from build123d import *

# Parameters (mm, degrees)
SKETCH2_R          = 1.8288
CUT_EXTRUDE1_DEPTH = 43.573973945


with BuildPart() as part:
    # Sketch1 → Revolve1 (revolve)
    with BuildSketch(Plane(origin=(0, 0, 0), x_dir=(1, 0, 0), z_dir=(0, 1, 0))):
        with BuildLine():
            Line((7.9629, -25.4), (44.45, -25.4))
            Line((44.45, -25.4), (44.45, 0))
            Line((44.45, 0), (46.99, 0))
            Line((46.99, 0), (58.473357526, 14.633973945))
            Line((58.473357526, 14.633973945), (48.488896002, -2.93998396))
            ThreePointArc((48.488896002, -2.93998396), (47.371046022, -5.678922959), (46.99, -8.612551998))
            Line((46.99, -8.612551998), (46.99, -27.94))
            Line((46.99, -27.94), (0, -27.94))
            Line((0, -27.94), (0, -15.24))
            Line((0, -15.24), (5.4229, -15.24))
            Line((5.4229, -15.24), (7.9629, -17.78))
            Line((7.9629, -17.78), (7.9629, -25.4))
        make_face()
    revolve(axis=Axis((0, 0, 0), (0, 0, 1)))

    # Sketch2 → Cut-Extrude1 (cut, through all)
    with BuildSketch(Plane.XY.offset(27.94)):
        with Locations((0, 16)):
            Circle(SKETCH2_R)
        with Locations((15.216904261, 4.94427191)):
            Circle(SKETCH2_R)
        with Locations((9.404564037, -12.94427191)):
            Circle(SKETCH2_R)
        with Locations((-9.404564037, -12.94427191)):
            Circle(SKETCH2_R)
        with Locations((-15.216904261, 4.94427191)):
            Circle(SKETCH2_R)
    extrude(amount=-CUT_EXTRUDE1_DEPTH, mode=Mode.SUBTRACT)


solid = part.part
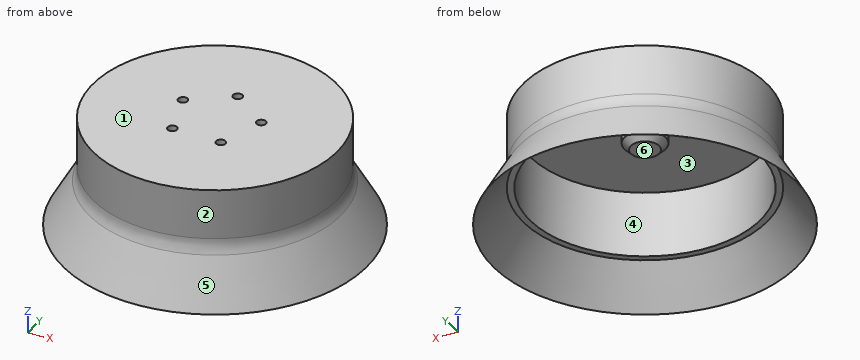
The model under review builds one solid part; all positions refer to its coordinate system, in mm. Face numbers are marked on the shaded views. A direction names the side the tool comes from. Give positions to 0.01 mm unless a question says otherwise; leave off trailing zeros. Loops run counter-clockwise (first coordinate to the right, second up) from the corner with the lowest first, then second, coordinate; pieces in that order, holes last. Notation, with made-up numbers: (63.5, -21) -> (97.5, -21) arc R10 cw to (97.5, -7) -> close; hole circle Ø5 at (81.5, 83). An arc over 180 degrees is marked (long way). Put each result on its own line as item: value. Start each with the question number.
1. Mouldability with a two-part tool opening along Y and no side actions: class the marked faces 1, 2, 3 and 4 as released by +Y, released by -Y, zero draft, split by the parting line, or undercut.
2. Wall thickness on probe 1 along Y at (x, z) = (0, 26); probe 2 along Z at (x, y) = (-25, 27); probe 3 along X at (y, z) = (-10, 9): over which ranges is each line inside the solid? List them lowest first.
3. Clearance check with flat-ended pins moving along their axes: P1, Ø6, axis at x = 2.5, z = -9.5, coming from the -Y side; P2, Ø5.5, axis at x = -1, y = 2, coming from the -Z side; P3, Ø4, axis at x = -7.5, y = -32.5, coming from the -Z side. State where each tip first meets the part, or that it passes through.
4. We need section A-A on x = 0. State the section outline as (y, z) points.
5. For the marked faces 5 and 6, list the 3-axis set-ups (+Z, -Z, +X, -X, +Y, -Y) from which the entire face can be reached by the end or side of a thin tool; tool diameter is ignored.
6. We need section B-B on y = 0. State the section outline as (x, z) points, then the cut area to 3 significant figures.
7. We need section C-C on z = -3. State the section outline as (x, y) points.
Determined:
1. face 1: zero draft
1. face 2: split by the parting line
1. face 3: undercut
1. face 4: undercut
2. probe 1: -46.99 to 14.17, 17.83 to 46.99
2. probe 2: 25.4 to 27.94
2. probe 3: -45.91 to -43.31, 43.31 to 45.91
3. P1: y = -57.21
3. P2: z = 15.24
3. P3: z = 25.4
4. outline: (-58.47, -14.63) -> (-46.99, 0) -> (-44.45, 0) -> (-44.45, 25.4) -> (-7.96, 25.4) -> (-7.96, 17.78) -> (-5.42, 15.24) -> (5.42, 15.24) -> (7.96, 17.78) -> (7.96, 25.4) -> (14.17, 25.4) -> (14.17, 27.94) -> (-46.99, 27.94) -> (-46.99, 8.61) arc R11.48 cw to (-48.49, 2.94) -> close; (17.83, 25.4) -> (44.45, 25.4) -> (44.45, 0) -> (46.99, 0) -> (58.47, -14.63) -> (48.49, 2.94) arc R11.48 cw to (46.99, 8.61) -> (46.99, 27.94) -> (17.83, 27.94) -> close
5. face 5: +Z
5. face 6: -Z
6. outline: (-58.47, -14.63) -> (-46.99, 0) -> (-44.45, 0) -> (-44.45, 25.4) -> (-7.96, 25.4) -> (-7.96, 17.78) -> (-5.42, 15.24) -> (5.42, 15.24) -> (7.96, 17.78) -> (7.96, 25.4) -> (44.45, 25.4) -> (44.45, 0) -> (46.99, 0) -> (58.47, -14.63) -> (48.49, 2.94) arc R11.48 cw to (46.99, 8.61) -> (46.99, 27.94) -> (-46.99, 27.94) -> (-46.99, 8.61) arc R11.48 cw to (-48.49, 2.94) -> close
6. area: 589 mm^2
7. outline: circle Ø103.73 at (0, 0); hole circle Ø98.69 at (0, 0)
